```python
from build123d import *

# Parameters (mm, degrees)
BOX024_W     = 59
BOX024_H     = 40
BOX024_DEPTH = 4
BOX002_W     = 86
BOX002_H     = 52
BOX002_DEPTH = 2.2
FILLET_R     = 4


with BuildPart() as display_cut:
    # Box024 → Box024 (new body)
    with BuildSketch(Plane(origin=(-26.5, -20.4, -18), x_dir=(1, 0, 0), z_dir=(0, 0, 1))):
        with Locations((29.5, 20)):
            Rectangle(BOX024_W, BOX024_H)
    extrude(amount=BOX024_DEPTH)


with BuildPart() as main_lid:
    # Box002 → Box002 (new body)
    with BuildSketch(Plane(origin=(-43, -26, -17.2), x_dir=(1, 0, 0), z_dir=(0, 0, 1))):
        with Locations((43, 26)):
            Rectangle(BOX002_W, BOX002_H)
    extrude(amount=BOX002_DEPTH)

    # Fillet
    fillet_edges = [main_lid.edges().sort_by_distance(p)[0] for p in [
        (-43, -26, -16.1),
        (-43, 26, -16.1),
        (43, -26, -16.1),
        (43, 26, -16.1),
    ]]
    fillet(fillet_edges, radius=FILLET_R)

    # Cut004: cut Display Cut
    add(display_cut.part, mode=Mode.SUBTRACT)


solid = main_lid.part
```
Source: CAD feature listing. Evaluate the final solid. Frame: model axes, mm. A direction names the side the tool comes from. Round coordinates to 2 decimals unless told otherwise and drop trailing zeros. Order: outer loops, then holes, each group sorted by start corner. A loop starts at its lowest first (then second) coordinate and runs counter-clockwise, first axis right, second up. Notation, with made-up numbers: (84, 53.5) -> (142, 53.5) arc R20 ccw to (142, 86.5) -> close; hole circle Ø1 at (23, 80.5). An arc over 180 degrees is marked (long way). One line per item, written item: value. Start each with the question number.
Q1. Access query for faces 1 (the flat face through (3, 19.6, -16)), 2 (the cylindrical face through (-41.859, -24.797, -16.085)). Directions: +Z, -Z, +X, -X, +Y, -Y. A direction counts if a zero-diameter tool reaches every point of the face in a straight line with its end or side. Return the directions, or none.
Q2. Section query C-C (z = -16.2). Return the cut outline in (x, y).
Q3. Draft query along Y for faces 3 (the cylindrical face through (-41.859, 24.797, -16.085)), 4 (the flat face through (32.5, -1, -16)), 5 (the cylindrical face through (41.797, -24.859, -16.085)), 6 (the flat face through (-43, 0, -16)). Return one class per face: pulls with the +Y half, pulls with the -Y half, needs draft (parallel to the pull), parting line crosses it, or undercut.
Q4. Pin query (flat end, axial travel): pin 1 (12 mm diameter, centred on x = 29, y = -5, fed in from -Z). Return the tip coordinate at first contact, or that it passes through.
Q5. Section query A-A (y = -19). Return the cut outline in (x, z).
Q6. Section query B-B (x = -25.5). Return the cut outline in (y, z).
Q7. Material intervals for probe 1 along X at (y, z) = (-19.5, -16.5); probe 2 along Y at (x, z) = (-20, -16); probe 3 along X at (y, z) = (23, -17), sorted ascending.
Findings below:
1. face 1: +Z, -Z
1. face 2: +Z, -Z, -X, -Y
2. outline: (-43, -22) arc R4 ccw to (-39, -26) -> (39, -26) arc R4 ccw to (43, -22) -> (43, 22) arc R4 ccw to (39, 26) -> (-39, 26) arc R4 ccw to (-43, 22) -> close; hole (-26.5, -20.4) -> (32.5, -20.4) -> (32.5, 19.6) -> (-26.5, 19.6) -> close
3. face 3: pulls with the +Y half
3. face 4: undercut
3. face 5: pulls with the -Y half
3. face 6: needs draft
4. pin 1: z = -17.2
5. outline: (-43, -17.2) -> (-26.5, -17.2) -> (-26.5, -15) -> (-43, -15) -> close; (32.5, -17.2) -> (43, -17.2) -> (43, -15) -> (32.5, -15) -> close
6. outline: (-26, -17.2) -> (-20.4, -17.2) -> (-20.4, -15) -> (-26, -15) -> close; (19.6, -17.2) -> (26, -17.2) -> (26, -15) -> (19.6, -15) -> close
7. probe 1: -43 to -26.5, 32.5 to 43
7. probe 2: -26 to -20.4, 19.6 to 26
7. probe 3: -42.87 to 42.87
